Input: dimensioned drawing with shaded views. Units: mm. Origin: part minimum x, y, z. Give positions to 0.01 mm unless a question says otherwise; leave off trailing zeros. Write each loop counter-clockwise with the first axis right and the second up, starting at its lowest first coordinate (ties: lowest second). Pieces come first, ordered by that corner, then holes. Notation, with made-up numbers: (79.25, 7) - (131.25, 7) arc R32 ccw to (131.25, 35) - close; hole circle Ø5 at (86.5, 24). An arc over 180 degrees is marked (long way). Answer as CSV lines item,"result".
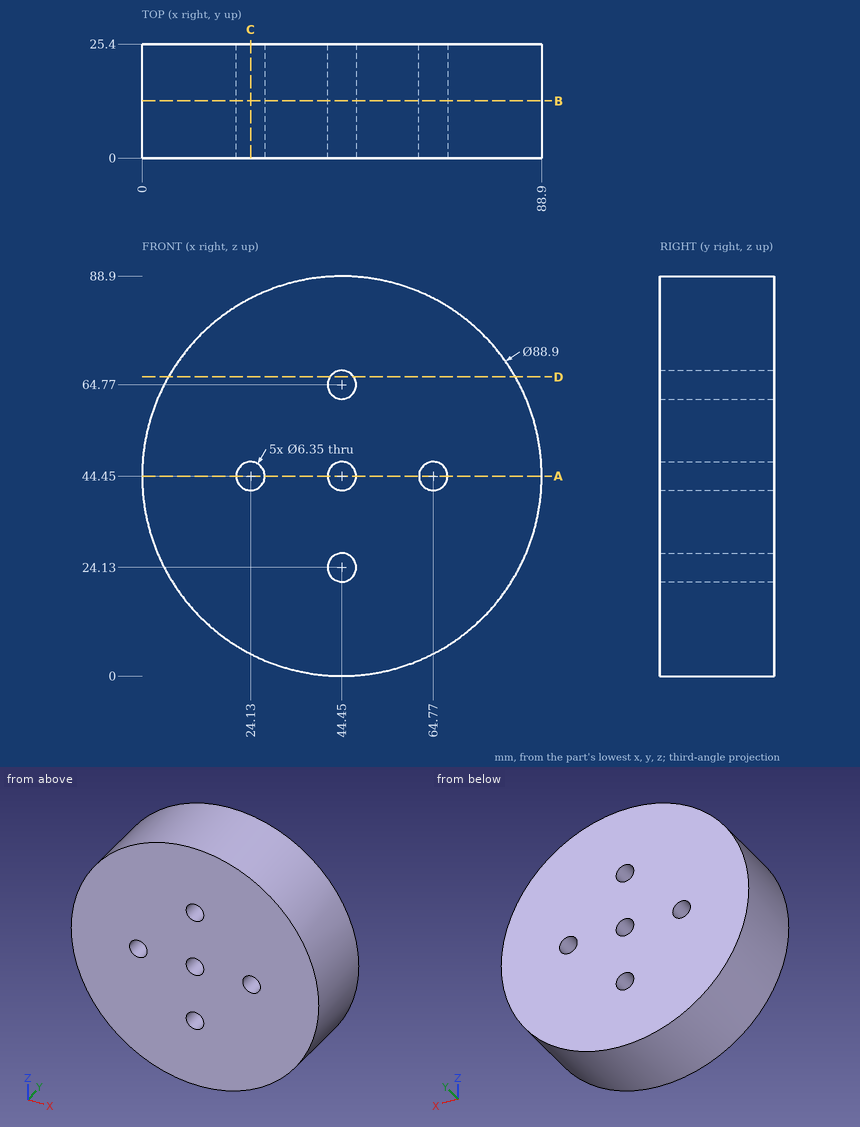
Item 1: Cut plane C-C on x = 24.13. Return the cut outline in (y, z) (3 decimals), plus the area to 3 significant figures.
The answers:
outline,"(0, 4.916) - (25.4, 4.916) - (25.4, 41.275) - (0, 41.275) - close; (0, 47.625) - (25.4, 47.625) - (25.4, 83.984) - (0, 83.984) - close"
area,"1,850 mm²"
Item 2: Cut plane D-D on z = 66.5. Return the cut outline in (x, y).
The answers:
outline,"(5.85, 0) - (41.79, 0) - (41.79, 25.4) - (5.85, 25.4) - close; (47.11, 0) - (83.05, 0) - (83.05, 25.4) - (47.11, 25.4) - close"
Item 3: Cut plane A-A on z = 44.45. Return the cut outline in (x, y) (3 decimals).
The answers:
outline,"(0, 0) - (20.955, 0) - (20.955, 25.4) - (0, 25.4) - close; (27.305, 0) - (41.275, 0) - (41.275, 25.4) - (27.305, 25.4) - close; (47.625, 0) - (61.595, 0) - (61.595, 25.4) - (47.625, 25.4) - close; (67.945, 0) - (88.9, 0) - (88.9, 25.4) - (67.945, 25.4) - close"
Item 4: Ray query, line 1 (Z direction, x = 44.45, y = 10.75) (3 decimals); line 2 (Z direction, x = 43.5, y = 7); line 3 (Z direction, x = 64.77, y = 9.5) (3 decimals). Return the intervals inside material, ascending. Write a range as from..to.
The answers:
line 1,"0..20.955, 27.305..41.275, 47.625..61.595, 67.945..88.9"
line 2,"0.01..21.1, 27.16..41.42, 47.48..61.74, 67.8..88.89"
line 3,"4.916..41.275, 47.625..83.984"
Item 5: Cut plane B-B on y = 12.75. Return the cut outline in (x, z) (3 decimals), plus the area to 3 significant figures.
The answers:
outline,"circle Ø88.9 at (44.45, 44.45); hole circle Ø6.35 at (24.13, 44.45); hole circle Ø6.35 at (44.45, 24.13); hole circle Ø6.35 at (44.45, 44.45); hole circle Ø6.35 at (44.45, 64.77); hole circle Ø6.35 at (64.77, 44.45)"
area,"6,050 mm²"
Item 6: Contact query for flat-ended pins moving along their axis: pin 1 (5 mm diameter, centred on x = 44.45, z = 64.77, fed in from +Y); pin 2 (6 mm diameter, centred on x = 49, y = 13, fed in from -Z); pin 3 (3 mm diameter, centred on x = 18.5, y = 14.5, fed in from +Z); pin 4 (4 mm diameter, centred on y = 12.5, z = 78, fed in from -X). Output: stop coordinate, or through.
The answers:
pin 1,"through"
pin 2,"z = 0.03"
pin 3,"z = 81.57"
pin 4,"x = 13.14"
